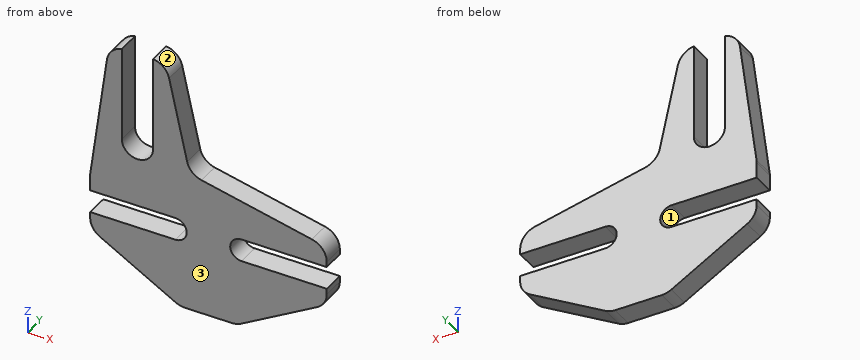
```python
from build123d import *

# Parameters (mm, degrees)
F1_DEPTH     = 12
F2_T1_DEPTH  = 12
F2_T3_DEPTH  = 54.7223945877
F2_T5_DEPTH  = 15.3186487605
F2_T7_DEPTH  = 41.0920435526
F2_T9_DEPTH  = 25.2174840277
F2_T11_DEPTH = 25.2174840277
F2_T13_DEPTH = 41.0920435526
F2_T15_DEPTH = 52.1292425836
F2_T17_DEPTH = 51.6983242764


# Not quite as in the source:
# - a fillet or chamfer that OpenCascade refuses, or shapes differently, is made with other operations: its cross-section is extruded or revolved along the edge and cut away or added


with BuildPart() as f1:
    # F0 (on Front) → F1 (new body)
    with BuildSketch(Plane.XZ):
        with BuildLine():
            Line((-52.5, 90), (-62.5, 15))
            Line((-62.5, 15), (-62.5, 6))
            Line((-62.5, 6), (-17.5, 6))
            ThreePointArc((-17.5, 6), (-11.5, 0), (-17.5, -6))
            Line((-17.5, -6), (-62.5, -6))
            Line((-62.5, -6), (-62.5, -15))
            Line((-62.5, -15), (-15, -42))
            Line((-15, -42), (15, -42))
            Line((15, -42), (62.5, -15))
            Line((62.5, -15), (62.5, -6))
            Line((62.5, -6), (17.5, -6))
            ThreePointArc((17.5, -6), (11.5, 0), (17.5, 6))
            Line((17.5, 6), (62.5, 6))
            Line((62.5, 6), (62.5, 16.9622953511))
            Line((62.5, 16.9622953511), (-9.86454105, 33.0051278665))
            Line((-9.86454105, 33.0051278665), (-22.5, 90))
            Line((-22.5, 90), (-29.25, 90))
            Line((-29.25, 90), (-29.25, 40))
            ThreePointArc((-29.25, 40), (-37.5, 31.75), (-45.75, 40))
            Line((-45.75, 40), (-45.75, 90))
            Line((-45.75, 90), (-52.5, 90))
        make_face()
    extrude(amount=F1_DEPTH)

    # F2: fillet of radius 10 on 9 edges, made by hand

    # F2_s2 → F2_t1 (join)
    with BuildSketch(Plane.XZ):
        with BuildLine():
            ThreePointArc((-3.6448495312, 31.6262554535), (-8.5515212037, 34.3181477128), (-11.243413463, 39.2248193853))
            Line((-11.243413463, 39.2248193853), (-9.86454105, 33.0051278665))
            Line((-9.86454105, 33.0051278665), (-3.6448495312, 31.6262554535))
        make_face()
    extrude(amount=F2_T1_DEPTH)

    # F2_s4 → F2_t3 (cut)
    with BuildSketch(Plane.XZ.offset(-21.3611972939)):
        with BuildLine():
            ThreePointArc((-53.62927012, 81.5304741001), (-51.0385819893, 87.0201735553), (-45.75, 90))
            Line((-45.75, 90), (-52.5, 90))
            Line((-52.5, 90), (-53.62927012, 81.5304741001))
        make_face()
    extrude(amount=F2_T3_DEPTH, mode=Mode.SUBTRACT)

    # F2_s6 → F2_t5 (cut)
    with BuildSketch(Plane.XZ.offset(-1.6593243803)):
        with BuildLine():
            ThreePointArc((-62.4122790068, 15.6579074488), (-62.478045652, 14.9985428246), (-62.5, 14.3362702479))
            Line((-62.5, 14.3362702479), (-62.5, 15))
            Line((-62.5, 15), (-62.4122790068, 15.6579074488))
        make_face()
    extrude(amount=F2_T5_DEPTH, mode=Mode.SUBTRACT)

    # F2_s8 → F2_t7 (cut)
    with BuildSketch(Plane.XZ.offset(-14.5460217763)):
        with BuildLine():
            ThreePointArc((-57.4416662495, -17.875263395), (-61.1433981308, -14.2106735867), (-62.5, -9.1815912895))
            Line((-62.5, -9.1815912895), (-62.5, -15))
            Line((-62.5, -15), (-57.4416662495, -17.875263395))
        make_face()
    extrude(amount=F2_T7_DEPTH, mode=Mode.SUBTRACT)

    # F2_s10 → F2_t9 (cut)
    with BuildSketch(Plane.XZ.offset(-6.6087420138)):
        with BuildLine():
            ThreePointArc((-12.3565031945, -42), (-14.9122104297, -41.6679036263), (-17.2981694439, -40.6936721056))
            Line((-17.2981694439, -40.6936721056), (-15, -42))
            Line((-15, -42), (-12.3565031945, -42))
        make_face()
    extrude(amount=F2_T9_DEPTH, mode=Mode.SUBTRACT)

    # F2_s12 → F2_t11 (cut)
    with BuildSketch(Plane.XZ.offset(-6.6087420138)):
        with BuildLine():
            ThreePointArc((17.2981694439, -40.6936721056), (14.9122104297, -41.6679036263), (12.3565031945, -42))
            Line((12.3565031945, -42), (15, -42))
            Line((15, -42), (17.2981694439, -40.6936721056))
        make_face()
    extrude(amount=F2_T11_DEPTH, mode=Mode.SUBTRACT)

    # F2_s14 → F2_t13 (cut)
    with BuildSketch(Plane.XZ.offset(-14.5460217763)):
        with BuildLine():
            ThreePointArc((62.5, -9.1815912895), (61.1433981308, -14.2106735867), (57.4416662495, -17.875263395))
            Line((57.4416662495, -17.875263395), (62.5, -15))
            Line((62.5, -15), (62.5, -9.1815912895))
        make_face()
    extrude(amount=F2_T13_DEPTH, mode=Mode.SUBTRACT)

    # F2_s16 → F2_t15 (cut)
    with BuildSketch(Plane.XZ.offset(-20.0646212918)):
        with BuildLine():
            ThreePointArc((54.6643961394, 18.6994069056), (60.2988448309, 15.1956815563), (62.5, 8.9364468344))
            Line((62.5, 8.9364468344), (62.5, 16.9622953511))
            Line((62.5, 16.9622953511), (54.6643961394, 18.6994069056))
        make_face()
    extrude(amount=F2_T15_DEPTH, mode=Mode.SUBTRACT)

    # F2_s18 → F2_t17 (cut)
    with BuildSketch(Plane.XZ.offset(-19.8491621382)):
        with BuildLine():
            ThreePointArc((-29.25, 90), (-23.7926014307, 87.4605787727), (-20.7815420039, 82.2485369039))
            Line((-20.7815420039, 82.2485369039), (-22.5, 90))
            Line((-22.5, 90), (-29.25, 90))
        make_face()
    extrude(amount=F2_T17_DEPTH, mode=Mode.SUBTRACT)


solid = f1.part
```
Check sheet for the modelled part. Datum: model origin and axes. Units: mm. Face numbers are marked on the shaded views. Give positions to 0.01 mm unless a question says otherwise; leave off trailing zeros. Order: outer loops, then holes, each group sorted by start corner. A loop starts at its lowest first (then second) coordinate and runs counter-clockwise, first axis right, second up. Notation, with made-up numbers: (49, 64.25) -> (54, 64.25) arc R32 cw to (54, 103.25) -> close; hole circle Ø5 at (36.25, -14.75). An arc over 180 degrees is marked (long way). Use CSV: the item, a comma, the result in double quotes. Start each with the question number.
1) Sectioned sample at C-C, the plane x = -24. Record the boundary of the cut face in (y, z), plus the area to 3 significant figures.
2) Sectioned sample at A-A, the plane z = 56.5. Record the boundary of the cut face in (x, y).
3) Go/stop test with flat-tipped pins: P1, Ø6, axis at x = 31.5, y = -3.5, coming from the -Z side; P2, Ø1, axis at y = -7.5, z = 17, coming from the +X side; P3, Ø6, axis at y = -6.5, z = 73, coming from the -X side. Record where each tip stops, or that it passes through.
4) Material ranges on line 1 (Z direction, x = -41.5, y = -4); line 2 (Z direction, x = -28, y = -9.5) (3 decimals); line 3 (X direction, y = -3, z = 61), recorded low to high. Write a range as from..to.
5) Sectioned sample at B-B, the plane y = -6.25. Record the boundary of the cut face in (x, z), plus the area to 3 significant figures.
6) Sectioned sample at D-D, the plane z = 0. Record the boundary of the cut face in (x, y).
7) Mould release check, pull along Z, two halves, no side actions. Record for the marked faces 1, 2 and 3: released by +Z, released by -Z, zero draft, split by the parting line, or undercut.
Recorded:
1,outline,"(-12, -36.88) -> (0, -36.88) -> (0, -6) -> (-12, -6) -> close; (-12, 6) -> (0, 6) -> (0, 87.65) -> (-12, 87.65) -> close"
1,area,"1,350 mm2"
2,outline,"(-56.97, -12) -> (-45.75, -12) -> (-45.75, 0) -> (-56.97, 0) -> close; (-29.25, -12) -> (-15.07, -12) -> (-15.07, 0) -> (-29.25, 0) -> close"
3,P1,"z = -34.33"
3,P2,"x = 59.04"
3,P3,"x = -55.17"
4,line 1,"-26.94..-6, 6..32.78"
4,line 2,"-34.611..-6, 6..89.755"
4,line 3,"-56.37..-45.75, -29.25..-16.07"
5,outline,"(-62.5, -9.18) arc R10 ccw to (-57.44, -17.88) -> (-17.3, -40.69) arc R10 ccw to (-12.36, -42) -> (12.36, -42) arc R10 ccw to (17.3, -40.69) -> (57.44, -17.88) arc R10 ccw to (62.5, -9.18) -> (62.5, -6) -> (17.5, -6) arc R6 cw to (17.5, 6) -> (62.5, 6) -> (62.5, 8.94) arc R10 ccw to (54.66, 18.7) -> (-3.64, 31.63) arc R10 cw to (-11.24, 39.22) -> (-20.78, 82.25) arc R10 ccw to (-29.25, 90) -> (-29.25, 40) arc R8.25 cw to (-45.75, 40) -> (-45.75, 90) arc R10 ccw to (-53.63, 81.53) -> (-62.41, 15.66) arc R10 ccw to (-62.5, 14.34) -> (-62.5, 6) -> (-17.5, 6) arc R6 cw to (-17.5, -6) -> (-62.5, -6) -> close"
5,area,"7,610 mm2"
6,outline,"(-11.5, -12) -> (11.5, -12) -> (11.5, 0) -> (-11.5, 0) -> close"
7,face 1,"undercut"
7,face 2,"released by +Z"
7,face 3,"zero draft"
